Read the model definition and answer for the solid it produces. Units are mm, in the model's axes. A direction names the side the tool comes from. Coordinates: 2 decimals unless noted, no trailing zeros. Write each loop counter-clockwise with the first axis right and the second up, starting at its lowest first coordinate (ties: lowest second). Pieces come first, ordered by that corner, then holes. Notation, with made-up numbers: (34.25, 51.5) -> (83.25, 51.5) arc R23 cw to (83.25, 60.5) -> close; hole circle Ø9 at (37, 11.5). An arc over 180 degrees is marked (long way). Answer in a Markdown table with one row per item. Add a question column.
Item 1: Which of the six approach directions +Z, -Z, +X, -X, +Y, -Y give full straight-line access (tool end or side, diameter ignored) to faces 4 (the face through (-82, 30, 20)), 5 (the face through (-80, 30, 20)), 6 (the face through (15, 30, 0))?
Item 2: Section B-B on z = 13.5 is taken. Write down the section's boundary in (x, y).
Item 3: Section D-D on y = 7.5 is taken. Write down the section's boundary in (x, z), then the cut area to 3 significant figures.
Item 4: For a pull along X with two mould halves and no side action, classify faces 1 (the face through (-0.98, 30.42, -1.03)), 2 (the face through (-61, 0, 41)), 3 (the face through (-0.97, 29.58, 40.98)) as +X half, -X half, draft (parallel to the pull), parting line (faces both ways), or undercut.
Item 5: Given pin 1 Ø23 at (x, y) = (11, 26) entering from +Z; pin 2 Ø10 at (y, z) = (40, 6.5) entering from +X; pin 3 Ø4 at (x, y) = (-25.5, 14.5) entering from -Z; pin 4 Ø1.9 at (x, y) = (-56.5, 45.5) entering from +Z, each flat-ended and moving along its own axis, determine where each tip first touches the part or whether it passes through.
Item 6: Section C-C on y = 30 is taken. Write down the section's boundary in (x, z), then the cut area to 3 significant figures.
Item 7: Section A-A on x = -98 is taken. Write down the section's boundary in (y, z), then the cut area to 3 significant figures.
Item 8: Straight lines are drawn through the part: line 1 (Y direction, x = -25.5, z = 40.95); line 2 (Y direction, x = 16, z = -1.2); line 3 (X direction, y = 16.5, z = 28.5). For each, find the intervals that lie inside material, in ascending order. Write a range as from..to.
```python
from build123d import *

# Parameters (mm, degrees)
SKETCH1_W                    = 30
SKETCH1_H                    = 60
BASE_FLANGE1_DEPTH           = 2
EDGE_FLANGE1_STRIP_W         = 12.8
EDGE_FLANGE1_STRIP_H         = 2
EDGE_FLANGE1_STRIP_CUT_DEPTH = 60
EDGE_FLANGE1_DEPTH           = 60
EDGE_FLANGE2_STRIP_W         = 12.8
EDGE_FLANGE2_STRIP_H         = 2
EDGE_FLANGE2_STRIP_CUT_DEPTH = 60
EDGE_FLANGE2_DEPTH           = 60
EDGE_FLANGE3_STRIP_W         = 12.8
EDGE_FLANGE3_STRIP_H         = 2
EDGE_FLANGE3_STRIP_CUT_DEPTH = 60
EDGE_FLANGE3_DEPTH           = 60
EDGE_FLANGE4_STRIP_W         = 12.8
EDGE_FLANGE4_STRIP_H         = 2
EDGE_FLANGE4_STRIP_CUT_DEPTH = 60
EDGE_FLANGE4_DEPTH           = 60
SKETCH22_R                   = 2.6
CUT_EXTRUDE1_DEPTH           = 133.800602408
SKETCH23_R                   = 11.5
SKETCH23_R_2                 = 1.6
CUT_EXTRUDE2_DEPTH           = 5


# Sheet-metal steps are written as plain solids
with BuildPart() as part:
    # Sketch1 → Base-Flange1 (new body)
    with BuildSketch(Plane.XY):
        with Locations((15, 30)):
            Rectangle(SKETCH1_W, SKETCH1_H)
    extrude(amount=-BASE_FLANGE1_DEPTH)

    # Edge-Flange1 strip (across the edge) → Edge-Flange1 strip cut (cut)
    with BuildSketch(Plane(origin=(-2, 60, 0), x_dir=(1, 0, 0), z_dir=(0, -1, 0))):
        with Locations((-3, -1)):
            Rectangle(EDGE_FLANGE1_STRIP_W, EDGE_FLANGE1_STRIP_H)
    extrude(amount=EDGE_FLANGE1_STRIP_CUT_DEPTH, mode=Mode.SUBTRACT)

    # Edge-Flange1 section (across the edge) → Edge-Flange1 (add)
    with BuildSketch(Plane(origin=(-2, 60, 0), x_dir=(1, 0, 0), z_dir=(0, -1, 0))):
        with BuildLine():
            Line((0, 1.4), (0, 40))
            Line((0, 40), (2, 40))
            Line((2, 40), (2, 1.4))
            ThreePointArc((2, 1.4), (2.410050506, 0.410050506), (3.4, 0))
            Line((3.4, 0), (3.4, -2))
            ThreePointArc((3.4, -2), (0.995836944, -1.004163056), (0, 1.4))
        make_face()
    extrude(amount=EDGE_FLANGE1_DEPTH)

    # Edge-Flange2 strip (across the edge) → Edge-Flange2 strip cut (cut)
    with BuildSketch(Plane(origin=(-2, 0, 42), x_dir=(0, 0, -1), z_dir=(0, 1, 0))):
        with Locations((-3, -1)):
            Rectangle(EDGE_FLANGE2_STRIP_W, EDGE_FLANGE2_STRIP_H)
    extrude(amount=EDGE_FLANGE2_STRIP_CUT_DEPTH, mode=Mode.SUBTRACT)

    # Edge-Flange2 section (across the edge) → Edge-Flange2 (add)
    with BuildSketch(Plane(origin=(-2, 0, 42), x_dir=(0, 0, -1), z_dir=(0, 1, 0))):
        with BuildLine():
            Line((0, 1.4), (0, 78))
            Line((0, 78), (2, 78))
            Line((2, 78), (2, 1.4))
            ThreePointArc((2, 1.4), (2.410050506, 0.410050506), (3.4, 0))
            Line((3.4, 0), (3.4, -2))
            ThreePointArc((3.4, -2), (0.995836944, -1.004163056), (0, 1.4))
        make_face()
    extrude(amount=EDGE_FLANGE2_DEPTH)

    # Edge-Flange3 strip (across the edge) → Edge-Flange3 strip cut (cut)
    with BuildSketch(Plane(origin=(-82, 0, 40), x_dir=(1, 0, 0), z_dir=(0, 1, 0))):
        with Locations((-3, -1)):
            Rectangle(EDGE_FLANGE3_STRIP_W, EDGE_FLANGE3_STRIP_H)
    extrude(amount=EDGE_FLANGE3_STRIP_CUT_DEPTH, mode=Mode.SUBTRACT)

    # Edge-Flange3 section (across the edge) → Edge-Flange3 (add)
    with BuildSketch(Plane(origin=(-82, 0, 40), x_dir=(1, 0, 0), z_dir=(0, 1, 0))):
        with BuildLine():
            Line((0, 1.4), (0, 40))
            Line((0, 40), (2, 40))
            Line((2, 40), (2, 1.4))
            ThreePointArc((2, 1.4), (2.410050506, 0.410050506), (3.4, 0))
            Line((3.4, 0), (3.4, -2))
            ThreePointArc((3.4, -2), (0.995836944, -1.004163056), (0, 1.4))
        make_face()
    extrude(amount=EDGE_FLANGE3_DEPTH)

    # Edge-Flange4 strip (across the edge) → Edge-Flange4 strip cut (cut)
    with BuildSketch(Plane(origin=(-82, 60, -2), x_dir=(0, 0, 1), z_dir=(0, -1, 0))):
        with Locations((-3, -1)):
            Rectangle(EDGE_FLANGE4_STRIP_W, EDGE_FLANGE4_STRIP_H)
    extrude(amount=EDGE_FLANGE4_STRIP_CUT_DEPTH, mode=Mode.SUBTRACT)

    # Edge-Flange4 section (across the edge) → Edge-Flange4 (add)
    with BuildSketch(Plane(origin=(-82, 60, -2), x_dir=(0, 0, 1), z_dir=(0, -1, 0))):
        with BuildLine():
            Line((0, 1.4), (0, 28))
            Line((0, 28), (2, 28))
            Line((2, 28), (2, 1.4))
            ThreePointArc((2, 1.4), (2.410050506, 0.410050506), (3.4, 0))
            Line((3.4, 0), (3.4, -2))
            ThreePointArc((3.4, -2), (0.995836944, -1.004163056), (0, 1.4))
        make_face()
    extrude(amount=EDGE_FLANGE4_DEPTH)

    # Sketch22 → Cut-Extrude1 (cut, through all)
    with BuildSketch(Plane(origin=(0, 0, -2), x_dir=(-1, 0, 0), z_dir=(0, 0, -1))):
        with Locations((-16, 45)):
            Circle(SKETCH22_R)
        with Locations((-16, 15)):
            Circle(SKETCH22_R)
        with Locations((98, 45)):
            Circle(SKETCH22_R)
        with Locations((98, 15)):
            Circle(SKETCH22_R)
    extrude(amount=-CUT_EXTRUDE1_DEPTH, mode=Mode.SUBTRACT)

    # Sketch23 → Cut-Extrude2 (cut)
    with BuildSketch(Plane.XY.offset(42)):
        with Locations((-41, 30)):
            Circle(SKETCH23_R)
        with Locations((-25.5, 45.5)):
            Circle(SKETCH23_R_2)
        with Locations((-25.5, 14.5)):
            Circle(SKETCH23_R_2)
        with Locations((-56.5, 14.5)):
            Circle(SKETCH23_R_2)
        with Locations((-56.5, 45.5)):
            Circle(SKETCH23_R_2)
    extrude(amount=-CUT_EXTRUDE2_DEPTH, mode=Mode.SUBTRACT)


solid = part.part
```
Results below:
| question | item | result |
|---|---|---|
| 1 | face 4 | +Z, -X, +Y, -Y |
| 1 | face 5 | -Z, +Y, -Y |
| 1 | face 6 | +Z, +X, +Y, -Y |
| 2 | outline | (-82, 0) -> (-80, 0) -> (-80, 60) -> (-82, 60) -> close; (-2, 0) -> (0, 0) -> (0, 60) -> (-2, 60) -> close |
| 3 | outline | (-110, -2) -> (-83.4, -2) arc R3.4 ccw to (-80, 1.4) -> (-80, 38.6) arc R1.4 cw to (-78.6, 40) -> (-3.4, 40) arc R1.4 cw to (-2, 38.6) -> (-2, 1.4) arc R3.4 ccw to (1.4, -2) -> (30, -2) -> (30, 0) -> (1.4, 0) arc R1.4 cw to (0, 1.4) -> (0, 38.6) arc R3.4 ccw to (-3.4, 42) -> (-78.6, 42) arc R3.4 ccw to (-82, 38.6) -> (-82, 1.4) arc R1.4 cw to (-83.4, 0) -> (-110, 0) -> close |
| 3 | area | 440 mm2 |
| 4 | face 1 | undercut |
| 4 | face 2 | draft |
| 4 | face 3 | +X half |
| 5 | pin 1 | stops at z = 40.37 |
| 5 | pin 2 | stops at x = 0 |
| 5 | pin 3 | stops at z = 40 |
| 5 | pin 4 | passes through |
| 6 | outline | (-110, -2) -> (-83.4, -2) arc R3.4 ccw to (-80, 1.4) -> (-80, 38.6) arc R1.4 cw to (-78.6, 40) -> (-52.5, 40) -> (-52.5, 42) -> (-78.6, 42) arc R3.4 ccw to (-82, 38.6) -> (-82, 1.4) arc R1.4 cw to (-83.4, 0) -> (-110, 0) -> close; (-29.5, 40) -> (-3.4, 40) arc R1.4 cw to (-2, 38.6) -> (-2, 1.4) arc R3.4 ccw to (1.4, -2) -> (30, -2) -> (30, 0) -> (1.4, 0) arc R1.4 cw to (0, 1.4) -> (0, 38.6) arc R3.4 ccw to (-3.4, 42) -> (-29.5, 42) -> close |
| 6 | area | 394 mm2 |
| 7 | outline | (0, -2) -> (12.4, -2) -> (12.4, 0) -> (0, 0) -> close; (17.6, -2) -> (42.4, -2) -> (42.4, 0) -> (17.6, 0) -> close; (47.6, -2) -> (60, -2) -> (60, 0) -> (47.6, 0) -> close |
| 7 | area | 99.2 mm2 |
| 8 | line 1 | y = 0..12.9, 16.1..43.9, 47.1..60 |
| 8 | line 2 | y = 0..12.4, 17.6..42.4, 47.6..60 |
| 8 | line 3 | x = -82..-80, -2..0 |
